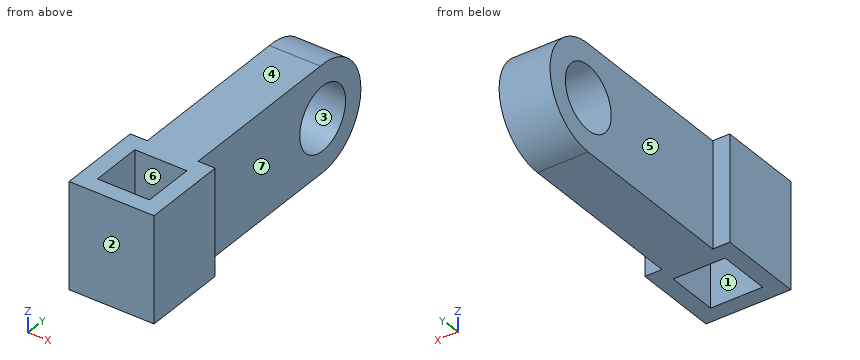
from build123d import *

# Parameters (mm, degrees)
SKETCH018_R             = 1.5
PAD012_DEPTH            = 2.4
BOX008_W                = 4
BOX008_H                = 5
BOX008_DEPTH            = 4
SKETCH019_W             = 2.45
SKETCH019_H             = 2.45
POCKET009_DEPTH         = 5.001
BODY005_PLACEMENT_ANGLE = 90


with BuildPart() as part:
    # Sketch018 → Pad012 (new body)
    with BuildSketch(Plane.XZ):
        with BuildLine():
            Line((-6, 5), (6, 5))
            ThreePointArc((6.150876, 0), (8.652014, 2.577748), (6, 5))
            Line((6.150876, 0), (-6, 0))
            Line((-6, 0), (-6, 5))
        make_face()
        with Locations((6.150876, 2.502276)):
            Circle(SKETCH018_R, mode=Mode.SUBTRACT)
    extrude(amount=PAD012_DEPTH)

    # Box008 → Box008 (join)
    with BuildSketch(Plane(origin=(-6, 0.8, 0), x_dir=(1, 0, 0), z_dir=(0, -1, 0))):
        with Locations((2, 2.5)):
            Rectangle(BOX008_W, BOX008_H)
    extrude(amount=BOX008_DEPTH)

    # Sketch019 (on Face13 of Box008) → Pocket009 (cut, through all)
    with BuildSketch(Plane(origin=(-6, 0.8, 5), x_dir=(-1, 0, 0), z_dir=(0, 0, 1))):
        with Locations((-2, 2)):
            Rectangle(SKETCH019_W, SKETCH019_H)
    extrude(amount=-POCKET009_DEPTH, mode=Mode.SUBTRACT)


with BuildPart() as part_1:
    # Body005 placement: moved
    add(part.part.moved(Location((40.3, -35.2, -10.6))).rotate(Axis((40.3, -35.2, -10.6), (0, 0, 1)), BODY005_PLACEMENT_ANGLE))


solid = part_1.part
Geometry: final body of the model. Coordinates: model frame, mm. Face numbers are marked on the shaded views. A direction names the side the tool comes from. Coordinates: 2 decimals unless noted, no trailing zeros. Loops run counter-clockwise (first coordinate to the right, second up) from the corner with the lowest first, then second, coordinate; pieces in that order, holes last. Notation, with made-up numbers: (-11, -12) - (45, -12) arc R30 ccw to (45, 11) - close; hole circle Ø3 at (79, 6). An arc over 180 degrees is marked (long way). One line per question, with ' | ' between items. Start each with the question number.
(1) Ray query, L1, parallel to Y at x = 40.8, z = -7.7 (3 decimals); L2, parallel to Y at x = 41.6, z = -6.9 (3 decimals); L3, parallel to Z at x = 40.8, y = -31. Return the intervals inside material, ascending. Write a range as from..to.
(2) Cut plane A-A on z = -7.5. Output: boundary loops of the cut face in (x, y) (3 decimals).
(3) Cut plane B-B on y = -39.25. Output: boundary loops of the cut face in (x, z) (3 decimals), and give its area (3 significant figures).
(4) First-contact query: pin 1 (1 mm diameter, centred on y = -32.5, z = -7.5, fed in from +X); pin 2 (1.5 mm diameter, centred on x = 41.5, z = -6, fed in from +Y); pin 3 (1.5 mm diameter, centred on y = -32.5, z = -9, fed in from -X). Flat tips, straight axial feed; report the tip coordinate or a pass-through.
(5) Cut plane D-D on z = -8.25. Output: boundary loops of the cut face in (x, y) (3 decimals), and give its area (3 significant figures).
(6) Reachability of the marked faces 5, 6 and 7 from +Z, -Z, +X, -X, +Y, -Y: full face, straight path, thin tool, end or side. Return the list, or none.
(7) Cut plane C-C on x = 40.65. Output: boundary loops of the cut face in (y, z) (3 decimals), and give its area (3 significant figures).
(8) Draft query along Y for the marked faces 1, 2, 3 and 4. Return one class per face: +Y half, -Y half, draft (parallel to the pull), parting line (faces both ways), or undercut.
Here are the results:
1) L1: -41.2..-40.425, -37.975..-30.495, -27.603..-26.579 | L2: -41.2..-40.425, -37.975..-29.952, -28.146..-26.852 | L3: -10.6..-5.6
2) outline: (39.5, -41.2) - (43.5, -41.2) - (43.5, -37.2) - (42.7, -37.2) - (42.7, -30.425) - (40.3, -30.425) - (40.3, -37.2) - (39.5, -37.2) - close; (40.3, -27.673) - (42.7, -27.673) - (42.7, -26.619) - (40.3, -26.619) - close; hole (40.275, -40.425) - (42.725, -40.425) - (42.725, -37.975) - (40.275, -37.975) - close
3) outline: (39.5, -10.6) - (40.275, -10.6) - (40.275, -5.6) - (39.5, -5.6) - close; (42.725, -10.6) - (43.5, -10.6) - (43.5, -5.6) - (42.725, -5.6) - close | area: 7.75 mm²
4) pin 1: x = 42.7 | pin 2: y = -26.94 | pin 3: x = 40.3
5) outline: (39.5, -41.2) - (43.5, -41.2) - (43.5, -37.2) - (42.7, -37.2) - (42.7, -30.541) - (40.3, -30.541) - (40.3, -37.2) - (39.5, -37.2) - close; (40.3, -27.557) - (42.7, -27.557) - (42.7, -26.551) - (40.3, -26.551) - close; hole (40.275, -40.425) - (42.725, -40.425) - (42.725, -37.975) - (40.275, -37.975) - close | area: 28.4 mm²
6) face 5: +Z, -Z, -X, +Y | face 6: +Z, -Z | face 7: +Z, -Z, +X, +Y
7) outline: (-41.2, -10.6) - (-40.425, -10.6) - (-40.425, -5.6) - (-41.2, -5.6) - close; (-37.975, -10.6) - (-29.049, -10.6) arc R2.502 ccw (long way) to (-29.2, -5.6) - (-37.975, -5.6) - close; hole circle Ø3 at (-29.049, -8.098) | area: 51.3 mm²
8) face 1: undercut | face 2: -Y half | face 3: undercut | face 4: draft
